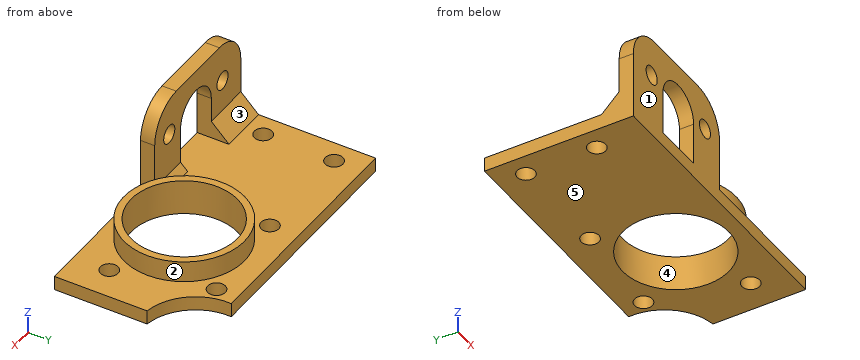
from build123d import *

# Parameters (mm, degrees)
BOX_W           = 80
BOX_H           = 42
BOX_DEPTH       = 4
SKETCH001_R     = 15
POCKET001_DEPTH = 4.001
SKETCH003_R     = 17
PAD_DEPTH       = 6
SKETCH004_R     = 15
POCKET003_DEPTH = 10.001
SKETCH005_R     = 2.5
POCKET004_DEPTH = 4.001
BOX001_W        = 40
BOX001_H        = 4
BOX001_DEPTH    = 25
SKETCH002_R     = 2.5781
POCKET002_DEPTH = 4.001
FILLET_R        = 10
FILLET001_R     = 10
CHAMFER_SIZE    = 5
CHAMFER001_SIZE = 2


with BuildPart() as pocket004:
    # Box → Box (new body)
    with BuildSketch(Plane(origin=(-768, 594, -534), x_dir=(1, 0, 0), z_dir=(0, 0, 1))):
        with Locations((40, 21)):
            Rectangle(BOX_W, BOX_H)
    extrude(amount=BOX_DEPTH)

    # Sketch001 → Pocket001 (cut, through all)
    with BuildSketch(Plane(origin=(-768, 594, -530), x_dir=(1, 0, 0), z_dir=(0, 0, 1))):
        with Locations((82, 41)):
            Circle(SKETCH001_R)
    extrude(amount=-POCKET001_DEPTH, mode=Mode.SUBTRACT)

    # Sketch003 → Pad (new body)
    with BuildSketch(Plane(origin=(-768, 594, -530), x_dir=(1, 0, 0), z_dir=(0, 0, 1))):
        with Locations((51, 19)):
            Circle(SKETCH003_R)
    extrude(amount=PAD_DEPTH)

    # Sketch004 → Pocket003 (cut, through all)
    with BuildSketch(Plane(origin=(-768, 594, -524), x_dir=(1, 0, 0), z_dir=(0, 0, 1))):
        with Locations((51, 19)):
            Circle(SKETCH004_R)
    extrude(amount=-POCKET003_DEPTH, mode=Mode.SUBTRACT)

    # Sketch005 → Pocket004 (cut, through all)
    with BuildSketch(Plane(origin=(-768, 594, -530), x_dir=(1, 0, 0), z_dir=(0, 0, 1))):
        with Locations((6.1, 34)):
            Circle(SKETCH005_R)
        with Locations((6.1, 14)):
            Circle(SKETCH005_R)
        with Locations((35.9, 34)):
            Circle(SKETCH005_R)
        with Locations((64, 36)):
            Circle(SKETCH005_R)
        with Locations((71, 10)):
            Circle(SKETCH005_R)
    extrude(amount=-POCKET004_DEPTH, mode=Mode.SUBTRACT)


with BuildPart() as chamfer001:
    # Box001 → Box001 (new body)
    with BuildSketch(Plane(origin=(-768, 594, -530), x_dir=(1, 0, 0), z_dir=(0, 0, 1))):
        with Locations((20, 2)):
            Rectangle(BOX001_W, BOX001_H)
    extrude(amount=BOX001_DEPTH)

    # Sketch002 → Pocket002 (cut, through all)
    with BuildSketch(Plane(origin=(-768, 598, -530), x_dir=(-1, 0, 0), z_dir=(0, 1, 0))):
        with Locations((-33.247, 14)):
            Circle(SKETCH002_R)
        with Locations((-8.5, 14)):
            Circle(SKETCH002_R)
        with BuildLine():
            ThreePointArc((-13.7, 12), (-20.85, 19.15), (-28, 12))
            Line((-28, 12), (-28, 0))
            Line((-28, 0), (-13.7, 0))
            Line((-13.7, 12), (-13.7, 0))
        make_face()
    extrude(amount=-POCKET002_DEPTH, mode=Mode.SUBTRACT)

    # Fillet
    fillet_edges = [chamfer001.edges().sort_by_distance(p)[0] for p in [
        (-728, 596, -505),
    ]]
    fillet(fillet_edges, radius=FILLET_R)

    # Fillet001
    fillet001_edges = [chamfer001.edges().sort_by_distance(p)[0] for p in [
        (-768, 596, -505),
    ]]
    fillet(fillet001_edges, radius=FILLET001_R)

    # Fusion: union Pocket004
    add(pocket004.part)

    # Chamfer
    chamfer_edges = [chamfer001.edges().sort_by_distance(p)[0] for p in [
        (-761.15, 598, -530),
    ]]
    chamfer(chamfer_edges, length=CHAMFER_SIZE)

    # Chamfer001
    chamfer001_edges = [chamfer001.edges().sort_by_distance(p)[0] for p in [
        (-734, 598, -530),
    ]]
    chamfer(chamfer001_edges, length=CHAMFER001_SIZE)


solid = chamfer001.part
Model file for the job. Use its own axes, mm. Face numbers are marked on the shaded views. A direction names the side the tool comes from. Give positions to 0.01 mm unless a question says otherwise; leave off trailing zeros. Write each loop counter-clockwise with the first axis right and the second up, starting at its lowest first coordinate (ties: lowest second). Pieces come first, ordered by that corner, then holes. Notation, with made-up numbers: (11.25, 8) - (50.25, 8) arc R11 ccw to (50.25, 22) - close; hole circle Ø9 at (80, -16). An arc over 180 degrees is marked (long way). Answer as CSV lines item,"result".
1. Drill centre lines: L1, parallel to Y at x = -761.9, z = -531.4; L2, parallel to X at y = 605, z = -531.5; L3, parallel to X at y = 596.3, z = -516. Where is each one in solid material? Low to high. Write a range as [from, to].
Responses:
L1,"y = [594, 605.5], [610.5, 625.5], [630.5, 636]"
L2,"x = [-768, -729.69], [-704.31, -699.29], [-694.71, -688]"
L3,"x = [-768, -762.08], [-756.92, -754.01], [-740.29, -737.33], [-732.17, -728]"
2. 3-axis set-ups, long thin cutter, end or side, ignore diameter. For the marked faces 1 and 2: which of +Z, -Z, +X, -X, +Y, -Y reach the whole face in a straight line?
Responses:
face 1,"+Z, -Z, +X, -X, -Y"
face 2,"+Z"
3. Band-saw the part on D-D (y = 608). Write the cut outline in (x, z), and give its area (3 significant figures).
Responses:
outline,"(-768, -534) - (-764.4, -534) - (-764.4, -530) - (-768, -530) - close; (-759.4, -534) - (-731.14, -534) - (-731.14, -524) - (-733.25, -524) - (-733.25, -530) - (-759.4, -530) - close; (-702.86, -534) - (-688, -534) - (-688, -530) - (-700.75, -530) - (-700.75, -524) - (-702.86, -524) - close"
area,"212 mm2"
4. Band-saw the part on C-C (z = -516). Write the cut outline in (x, y).
Responses:
outline,"(-768, 594) - (-762.08, 594) - (-762.08, 598) - (-768, 598) - close; (-756.92, 594) - (-754.01, 594) - (-754.01, 598) - (-756.92, 598) - close; (-740.29, 594) - (-737.33, 594) - (-737.33, 598) - (-740.29, 598) - close; (-732.17, 594) - (-728, 594) - (-728, 598) - (-732.17, 598) - close"
5. Band-saw the part on A-A (y = 613). Write the cut outline in (x, z), and give its area (3 significant figures).
Responses:
outline,"(-768, -534) - (-732, -534) - (-732, -524) - (-734, -524) - (-734, -530) - (-768, -530) - close; (-702, -534) - (-688, -534) - (-688, -530) - (-700, -530) - (-700, -524) - (-702, -524) - close"
area,"224 mm2"
6. Band-saw the part on B-B (x = -747.15). Write the cut outline in (y, z), and give its area (3 significant figures).
Responses:
outline,"(594, -534) - (636, -534) - (636, -530) - (594, -530) - close; (594, -510.85) - (598, -510.85) - (598, -505) - (594, -505) - close"
area,"191 mm2"
7. Pin check, flat tips, straight feed: pin 1 (3 mm diameter, centred on x = -732.1, y = 628, fed in from -Z); pin 2 (8 mm diameter, centred on x = -697, y = 604, fed in from +Z); pin 3 (8 mm diameter, centred on x = -757.5, z = -514, fed in from +Y); pin 4 (4.5 mm diameter, centred on y = 598, z = -526.5, fed in from +X). Stop position of each tip, or through.
Responses:
pin 1,"passes through"
pin 2,"stops at z = -530"
pin 3,"stops at y = 598"
pin 4,"stops at x = -705.76"
8. Two-plate mould, pull along Y, no slides. Class the marked faces 3, 4 and 5: +Y half, -Y half, draft (parallel to the pull), parting line (faces both ways), or undercut.
Responses:
face 3,"+Y half"
face 4,"undercut"
face 5,"draft"
